Geometry check sheet. Reference: the model listing, model coordinates, mm. Face numbers are marked on the shaded views. A direction names the side the tool comes from. Give positions to 0.01 mm unless a question says otherwise; leave off trailing zeros. Order: outer loops, then holes, each group sorted by start corner. A loop starts at its lowest first (then second) coordinate and runs counter-clockwise, first axis right, second up. Notation, with made-up numbers: M 34,48.25 L 60,48.25 A18 cw 60,61.25 Z; hole C 57.5,60 d10. An arc over 180 degrees is marked long. Put each result on its own line as item: value. Start each with the question number.
Q1. Mould release check, pull along Z, two halves, no side actions. Record for the marked faces 3, 4 and 5: +Z half, -Z half, draft (parallel to the pull), parting line (faces both ways), or undercut.
Q2. Go/stop test with flat-tipped pins: pin 1 (8 mm diameter, centred on x = -18.5, y = 7.5, fed in from +Z); pin 2 (12 mm diameter, centred on x = -15, z = 1, fed in from -Y); pin 3 (3.5 mm diameter, centred on x = 0.5, z = -0.5, fed in from +Y). Record where each tip stops, or that it passes through.
Q3. Access from +Z, -Z, +X, -X, +Y, -Y to the whole of each face (thin tool, end or side, straight path). Record for the marked faces 1 and 2.
Q4. Section check D-D on z = -6. Record the cut outline in (x, y), then the cut area to 3 significant figures.
Q5. Material ranges on L1, parallel to Z at x = -20, y = 2.5; L2, parallel to Y at x = -5.5, z = -6.25; L3, parallel to X at y = 5.25, z = -8, recorded low to high.
Q6. Section check B-B on x = -7.5. Record the cut outline in (y, z).
Q7. Section check A-A on z = 0. Record the cut outline in (x, y).
Q8. Section check C-C on y = 8.75. Record the cut outline in (x, z).
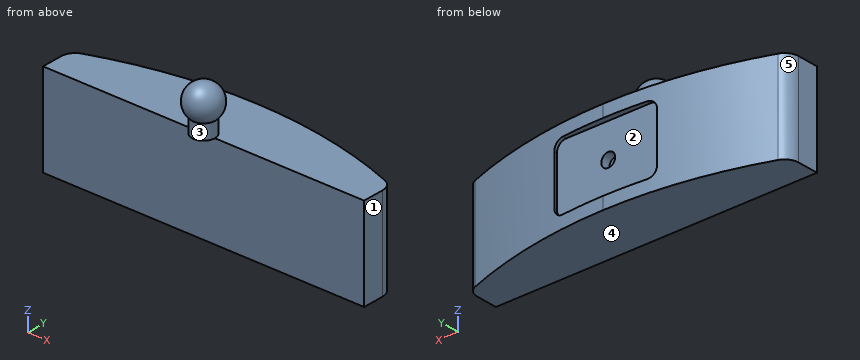
```python
from build123d import *

# Parameters (mm, degrees)
SKETCH1_W           = 69.3
SKETCH1_H           = 19.8
BOSS_EXTRUDE1_DEPTH = 13.3
CUT_EXTRUDE1_DEPTH  = 48.412254857
CUT_EXTRUDE2_DEPTH  = 3
SKETCH5_R           = 1.5
CUT_EXTRUDE3_DEPTH  = 2
FILLET1_R           = 3


with BuildPart() as part:
    # Sketch1 → Boss-Extrude1 (new body)
    with BuildSketch(Plane(origin=(0, 0, 0), x_dir=(1, 0, 0), z_dir=(0, 1, 0))):
        Rectangle(SKETCH1_W, SKETCH1_H)
    extrude(amount=BOSS_EXTRUDE1_DEPTH)

    # Sketch2 → Revolve1 (revolve)
    with BuildSketch(Plane(origin=(0, 0, 0), x_dir=(1, 0, 0), z_dir=(0, 1, 0))):
        with BuildLine():
            Line((2.465, -9.9), (2.465, -13.12))
            ThreePointArc((2.465, -13.12), (3.467767545, -17.211295036), (0, -19.602701751))
            Line((0, -19.602701751), (0, -9.9))
            Line((0, -9.9), (2.465, -9.9))
        make_face()
    revolve(axis=Axis((0, 0, 0), (0, 0, 1)))

    # Sketch3 → Cut-Extrude1 (cut, through all)
    with BuildSketch(Plane(origin=(0, 0, -9.9), x_dir=(-1, 0, 0), z_dir=(0, 0, -1))):
        with BuildLine():
            Line((-34.65, 13.3), (-34.65, 6.65))
            ThreePointArc((-34.65, 6.65), (-17.641180346, 11.622466932), (3.46e-07, 13.3))
            Line((3.46e-07, 13.3), (-34.65, 13.3))
        make_face()
        with BuildLine():
            ThreePointArc((3.46e-07, 13.3), (17.641180686, 11.622466867), (34.65, 6.65))
            Line((34.65, 6.65), (34.65, 13.3))
            Line((34.65, 13.3), (3.46e-07, 13.3))
        make_face()
    extrude(amount=-CUT_EXTRUDE1_DEPTH, mode=Mode.SUBTRACT)

    # Sketch4 → Cut-Extrude2 (cut)
    with BuildSketch(Plane(origin=(0, 15, 0), x_dir=(1, 0, 0), z_dir=(0, 1, 0))):
        with BuildLine():
            Line((-9.1, -7.25), (9.1, -7.25))
            ThreePointArc((9.1, -7.25), (10.514213562, -6.664213562), (11.1, -5.25))
            Line((11.1, -5.25), (11.1, 5.25))
            ThreePointArc((11.1, 5.25), (10.514213562, 6.664213562), (9.1, 7.25))
            Line((9.1, 7.25), (-9.1, 7.25))
            ThreePointArc((-9.1, 7.25), (-10.514213562, 6.664213562), (-11.1, 5.25))
            Line((-11.1, 5.25), (-11.1, -5.25))
            ThreePointArc((-11.1, -5.25), (-10.514213562, -6.664213562), (-9.1, -7.25))
        make_face()
    extrude(amount=-CUT_EXTRUDE2_DEPTH, mode=Mode.SUBTRACT)

    # Sketch5 → Cut-Extrude3 (cut)
    with BuildSketch(Plane(origin=(0, 12, 0), x_dir=(1, 0, 0), z_dir=(0, 1, 0))):
        with Locations(Location((0, 0, 0), (0, 0, 270))):
            Circle(SKETCH5_R)
    extrude(amount=-CUT_EXTRUDE3_DEPTH, mode=Mode.SUBTRACT)

    # Fillet1
    fillet1_edges = [part.edges().sort_by_distance(p)[0] for p in [
        (34.65, 6.65, 0),
        (-34.65, 6.65, 0),
    ]]
    fillet(fillet1_edges, radius=FILLET1_R)


solid = part.part
```
Results found:
1. face 3: undercut
1. face 4: -Z half
1. face 5: draft
2. pin 1: stops at z = 9.9
2. pin 2: stops at y = 0
2. pin 3: stops at y = 12
3. face 1: +Z, -Z, +X, +Y, -Y
3. face 2: +Y
4. outline: M -34.65,0 L 34.65,0 L 34.65,4.59 A3 ccw 32.7,7.4 A93.6 ccw 10.95,12.66 L 10.95,12 L -10.95,12 L -10.95,12.66 A93.6 ccw -32.7,7.4 A3 ccw -34.65,4.59 Z
4. area: 745 mm^2
5. L1: z = -9.9 to 9.9
5. L2: y = 0 to 12
5. L3: x = -34.58 to 34.58
6. outline: M 0,-9.9 L 13,-9.9 L 13,-7.25 L 12,-7.25 L 12,7.25 L 13,7.25 L 13,9.9 L 0,9.9 Z
7. outline: M -34.65,0 L 34.65,0 L 34.65,4.59 A3 ccw 32.7,7.4 A93.6 ccw 11.1,12.64 L 11.1,12 L 1.5,12 L 1.5,10 L -1.5,10 L -1.5,12 L -11.1,12 L -11.1,12.64 A93.6 ccw -32.7,7.4 A3 ccw -34.65,4.59 Z
8. outline: M -28.83,-9.9 L 28.83,-9.9 L 28.83,9.9 L -28.83,9.9 Z
